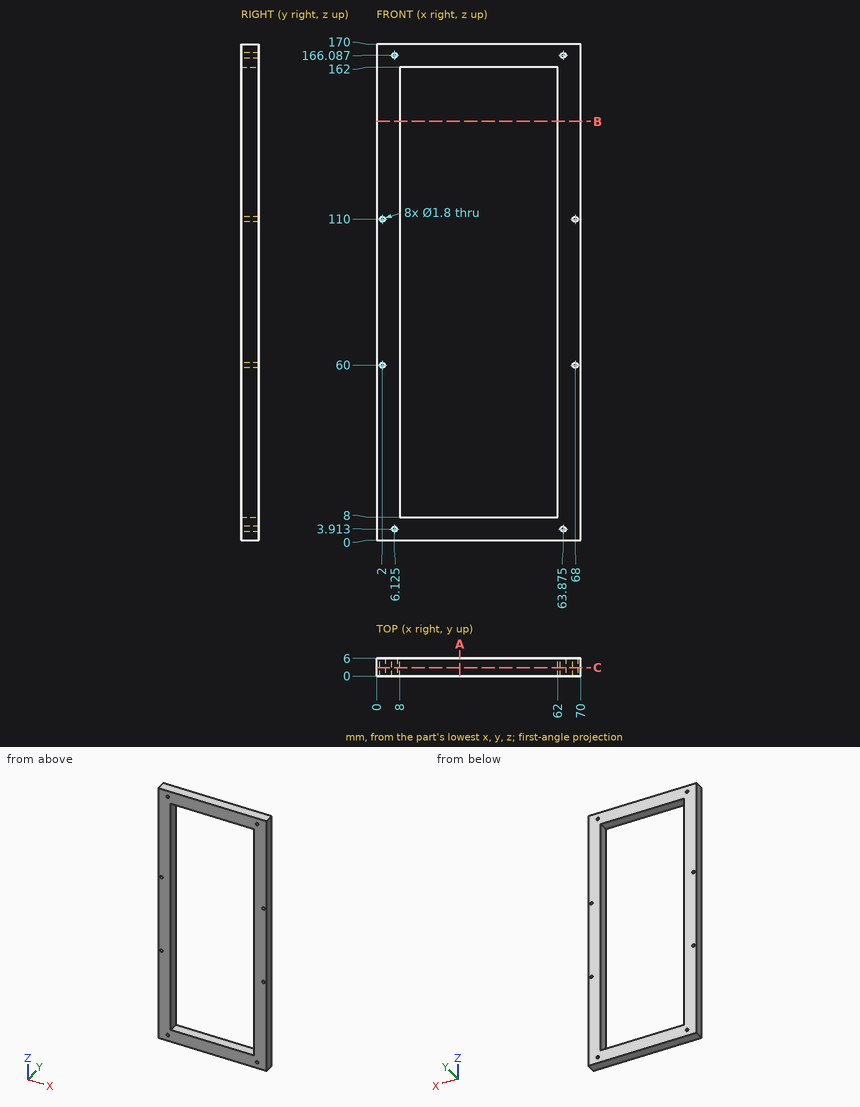
Input: dimensioned drawing with shaded views. Units: mm. Origin: part minimum x, y, z. Give positions to 0.01 mm unless a question says otherwise; leave off trailing zeros. Order: outer loops, then holes, each group sorted by start corner. A loop starts at its lowest first (then second) coordinate and runs counter-clockwise, first axis right, second up. Notation, with made-up numbers: (68, -19.75) -> (87, -19.75) arc R18 ccw to (87, 3.25) -> close; hole circle Ø3 at (10, 67.25). An arc over 180 degrees is marked (long way). Answer as a JSON object with one key per item and string values.
Q1. Section B-B (z = 143.5). Output: boundary loops of the cut face in (x, y).
Entries:
{"outline": "(0, 0) -> (8, 0) -> (8, 6) -> (0, 6) -> close; (62, 0) -> (70, 0) -> (70, 6) -> (62, 6) -> close"}
Q2. Section A-A (x = 28.5). Output: boundary loops of the cut face in (y, z).
Entries:
{"outline": "(0, 0) -> (6, 0) -> (6, 8) -> (0, 8) -> close; (0, 162) -> (6, 162) -> (6, 170) -> (0, 170) -> close"}
Q3. First-contact query: pin 1 (1.8 mm diameter, centred on y = 3, z = 76, fed in from -X). Flat tip, straight axial feed; report the tip coordinate or a pass-through.
Entries:
{"pin 1": "stops at x = 0"}
Q4. Material intervals for probe 1 along Z at (x, y) = (2, 2.1); probe 2 along X at (y, z) = (4.05, 60); probe 3 along X at (y, z) = (4.5, 21), sorted ascending.
Entries:
{"probe 1": "z = 0 to 59.1, 60.9 to 109.1, 110.9 to 170", "probe 2": "x = 0 to 1.1, 2.9 to 8, 62 to 67.1, 68.9 to 70", "probe 3": "x = 0 to 8, 62 to 70"}
Q5. Section C-C (y = 2.9). State how many separate pieces and enclosed holes the cut face has, plus the area to 3 significant figures.
Entries:
{"separate pieces": "1", "enclosed holes": "9", "area": "3,560 mm^2"}
